The figure shows three views and two pictorial views of one solid part (mm, origin at its lowest corner). Answer the questions. Coordinates: 2 decimals unless noted, no trailing zeros. Write each loop counter-clockwise with the first axis right and the second up, starting at its lowest first coordinate (ties: lowest second). Pieces come first, ordered by that corner, then holes. Notation, with made-up numbers: M 12.25,32 L 26.25,32 A32 cw 26.25,62 Z; hole C 40,55 d6. An arc over 180 degrees is marked long. Answer as CSV lines item,"result".
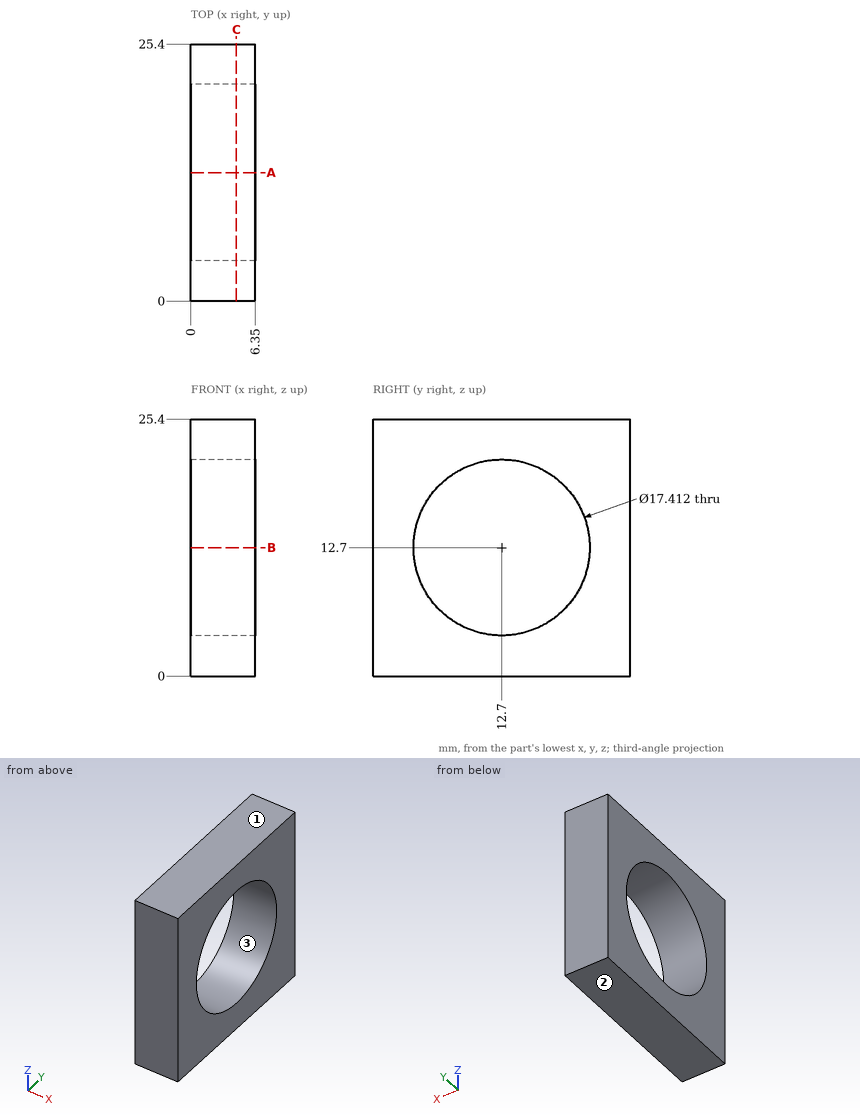
Q1. Straight lines are drawn through the part: line 1 (Y direction, x = 2.5, z = 12.7); line 2 (Z direction, x = 0.5, y = 19); line 3 (Z direction, x = 5.25, y = 6.25). For each, find the intervals that lie inside material, in ascending order.
Output:
line 1,"0 to 3.99, 21.41 to 25.4"
line 2,"0 to 6.69, 18.71 to 25.4"
line 3,"0 to 6.85, 18.55 to 25.4"
Q2. The mould has two halves that part along Z. Classify the marked faces 1, 2 and 3: pulls with the +Z half, pulls with the -Z half, needs draft (parallel to the pull), parting line crosses it, or undercut.
Output:
face 1,"pulls with the +Z half"
face 2,"pulls with the -Z half"
face 3,"undercut"
Q3. Find section C-C (x = 4.5). Give the vertices of the cut face in (y, z).
Output:
outline,"M 0,0 L 25.4,0 L 25.4,25.4 L 0,25.4 Z; hole C 12.7,12.7 d17.41"
Q4. Find section A-A (y = 12.7). Give the vertices of the cut face in (x, z).
Output:
outline,"M 0,0 L 6.35,0 L 6.35,3.99 L 0,3.99 Z; M 0,21.41 L 6.35,21.41 L 6.35,25.4 L 0,25.4 Z"
